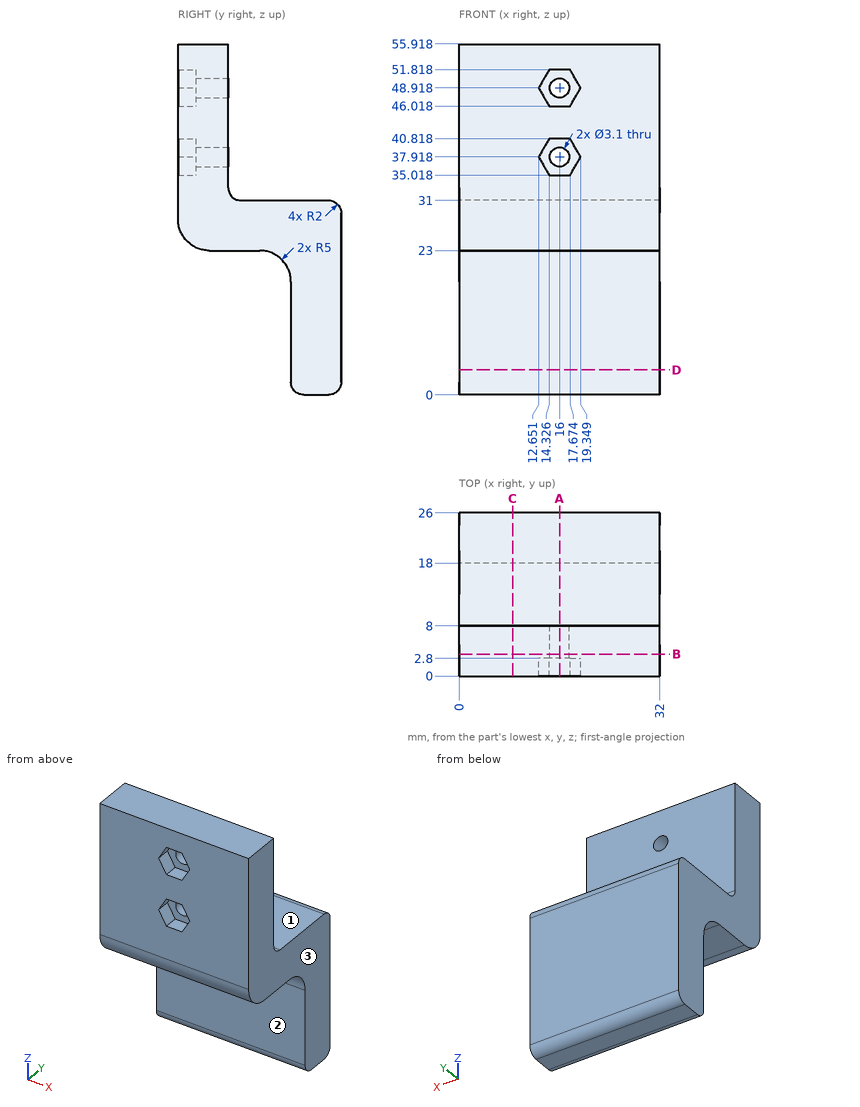
Print and shaded views of the part. All mm, measured from the part's lowest x, y and z. A direction names the side the tool comes from. Coordinates: 2 decimals unless noted, no trailing zeros. Order: outer loops, then holes, each group sorted by start corner. A loop starts at its lowest first (then second) coordinate and runs counter-clockwise, first axis right, second up. Notation, with made-up numbers: (-9, -10.75) - (2, -10.75) arc R4 ccw to (2, -6.75) - close; hole circle Ø11 at (-2, 74). An arc over 180 degrees is marked (long way). Return JSON: item names as keys, results as strings. Group by question number.
Item 1: Pin check, flat tips, straight feed: pin 1 (7 mm diameter, centred on x = 18, z = 40, fed in from +Y); pin 2 (3 mm diameter, centred on x = 16.5, y = 2, fed in from -Z); pin 3 (1.5 mm diameter, centred on x = 10.5, y = 19, fed in from -Z); pin 4 (8 mm diameter, centred on y = 21, z = 36.5, fed in from -X). Stop position of each tip, or through.
Item 2: Cut at D-D (z = 4). List the corners of the cut face in (x, y), plus the area to 3 significant figures.
Item 3: Drill centre lines: probe 1 along Z at (x, y) = (16, 5.9); probe 2 along Y at (x, z) = (9.5, 41); probe 3 along Z at (x, y) = (29, 20.75). Where is each one in solid material? Low to high. Write a range as from..to.
Item 4: Cut at A-A (x = 16). State how many separate pieces and enclosed holes the cut face has, plus the area to 3 significant figures.
Item 5: Cut at C-C (x = 8.5). List the corners of the cut face in (y, z).
Item 6: Which spindle directions (+Z, -Z, +X, -X, +Y, -Y) get a long thin tool onto all of the face, cutting with end or side? Do the marked faces 1, 2 and 3. Say none if no direction does.
Item 7: Cut at B-B (y = 3.5). List the corners of the cut face in (x, z), plus the area to 3 significant figures.
Check values:
{
 "1": {"pin 1": "stops at y = 8", "pin 2": "stops at z = 23.23", "pin 3": "stops at z = 0.02", "pin 4": "passes through"},
 "2": {"outline": "(0, 18) - (32, 18) - (32, 26) - (0, 26) - close", "area": "256 mm2"},
 "3": {"probe 1": "z = 23..36.37, 39.47..47.37, 50.47..55.92", "probe 2": "y = 0..8", "probe 3": "z = 0..31"},
 "4": {"separate pieces": "3", "enclosed holes": "0", "area": "525 mm2"},
 "5": {"outline": "(0, 28) arc R5 ccw to (5, 23) - (13, 23) arc R5 cw to (18, 18) - (18, 2) arc R2 ccw to (20, 0) - (24, 0) arc R2 ccw to (26, 2) - (26, 29) arc R2 ccw to (24, 31) - (10, 31) arc R2 cw to (8, 33) - (8, 55.92) - (0, 55.92) - close"},
 "6": {"face 1": "+Z, +X, -X, +Y", "face 2": "-Z, +X, -X, -Y", "face 3": "+Z, -Z, +X, +Y, -Y"},
 "7": {"outline": "(0, 23.23) - (32, 23.23) - (32, 55.92) - (0, 55.92) - close; hole circle Ø3.1 at (16, 37.92); hole circle Ø3.1 at (16, 48.92)", "area": "1,030 mm2"}
}
